Read the model definition and answer for the solid it produces. Units are mm, in the model's axes. A direction names the side the tool comes from. Give positions to 0.01 mm unless a question says otherwise; leave off trailing zeros. Write each question's results on one line, items separated by ' | '.
Autodesk Inventor part; units mm, degrees
ref_plane "YZ Plane" through (0, 0, 0) normal (1, 0, 0) x (0, 1, 0)
ref_plane "XZ Plane" through (0, 0, 0) normal (0, 1, 0) x (-1, 0, 0)
ref_plane "XY Plane" through (0, 0, 0) normal (0, 0, 1) x (1, 0, 0)
sketch "Sketch1" plane through (0, 0, 0) normal (0, 0, 1) x (1, 0, 0)
  line L0 (-63.5, -63.5) -> (63.5, -63.5)
  line L1 (63.5, -63.5) -> (63.5, 63.5)
  line L2 (63.5, 63.5) -> (-63.5, 63.5)
  line L3 (-63.5, 63.5) -> (-63.5, -63.5)
  line L4 (-63.5, -63.5) -> (63.5, 63.5) construction
  line L5 (63.5, -63.5) -> (-63.5, 63.5) construction
  circle A0 centre (0, 0) radius 47.5
  circle A1 centre (0, 0) radius 38.77
  circle A2 centre (0, 0) radius 40.635
  dimension "d0" = 127
  dimension "d1" = 127
  dimension "d2" = 95
  dimension "d3" = 77.54
  dimension "d4" = 81.27
extrude "Extrusion1" add sketch "Sketch1" against normal blind 9.525 contours L3 L2 L1 L0 | A0 | A2
extrude "Extrusion2" cut sketch "Sketch1" against normal blind 4.7625 contours A0
extrude "Extrusion3" cut sketch "Sketch1" against normal blind 5.1594 contours A2
sketch "Sketch2" plane through (0, 0, -9.525) normal (0, 0, -1) x (-1, 0, 0)
  circle A0 centre (0, 0) radius 38.77
  circle A1 centre (0, 0) radius 38.1
  circle A2 centre (0, 0) radius 48.0219
  dimension "d11" = 76.2
  dimension "d12" = 96.0438
extrude "Extrusion4" cut sketch "Sketch2" against normal blind 0.7937 contours A2
sketch "Sketch3" plane through (0, 0, 0) normal (0, 0, 1) x (1, 0, 0)
  line L0 (-63.5, -63.5) -> (63.5, -63.5)
  line L1 (63.5, -63.5) -> (63.5, 63.5)
  line L2 (63.5, 63.5) -> (-63.5, 63.5)
  line L3 (-63.5, 63.5) -> (-63.5, -63.5)
  circle A0 centre (0, 0) radius 47.5
  circle A1 centre (0, 0) radius 53.975
  dimension "d16" = 107.95
extrude "Extrusion5" cut sketch "Sketch3" against normal blind 3.175 contours L3 L2 L1 L0
fillet "Fillet1" radius 3.175 1 edges at (-53.975, 0, -3.175)
properties part number "Swerve Pre Baseplate"
(1) For faces 5 (the face through (10.41, -46.88, -9.13)), 6 (the face through (63.5, -1, -6)), 7 (the face through (38.759, 12.206, -4.958)), determine the directions among +Z, -Z, +X, -X, +Y, -Y from which every point of the face is accessible in a straight line to the end or side of a thin tool.
Conclusion:
face 5: -Z | face 6: +Z, -Z, +X, +Y, -Y | face 7: +Z
(2) Consider probe 1 along Y at (x, z) = (0, -4); probe 2 along Y at (x, z) = (0, -5) (3 decimals); probe 3 along Z at (x, y) = (36.5, 14). Determine where each line is inside the solid, lowest interval first. Write a range as [from, to].
Conclusion:
probe 1: [-63.5, -47.5], [47.5, 63.5] | probe 2: [-63.5, -40.635], [40.635, 63.5] | probe 3: [-8.73, -5.16]
(3) The mould has two halves that part along X. Classify faces 1 (the face through (-63.5, 1, -6)), 2 (the face through (-3, 39, -8.731)), 3 (the face through (1, 63.5, -6)), 4 (the face through (-10.3, -46.37, -2.35)): pulls with the +X half, pulls with the -X half, needs draft (parallel to the pull), parting line crosses it, or undercut.
Conclusion:
face 1: pulls with the -X half | face 2: undercut | face 3: needs draft | face 4: undercut
(4) Each of these flat-tipped pins is pushed along its axis until it touches: pin 1 (1 mm diameter, centred on x = -40, y = -7, fed in from -Z); pin 2 (1 mm diameter, centred on x = 40, y = -13.5, fed in from +Z). Where does it stop, or does it pass through?
Conclusion:
pin 1: z = -8.73 | pin 2: z = -4.76
